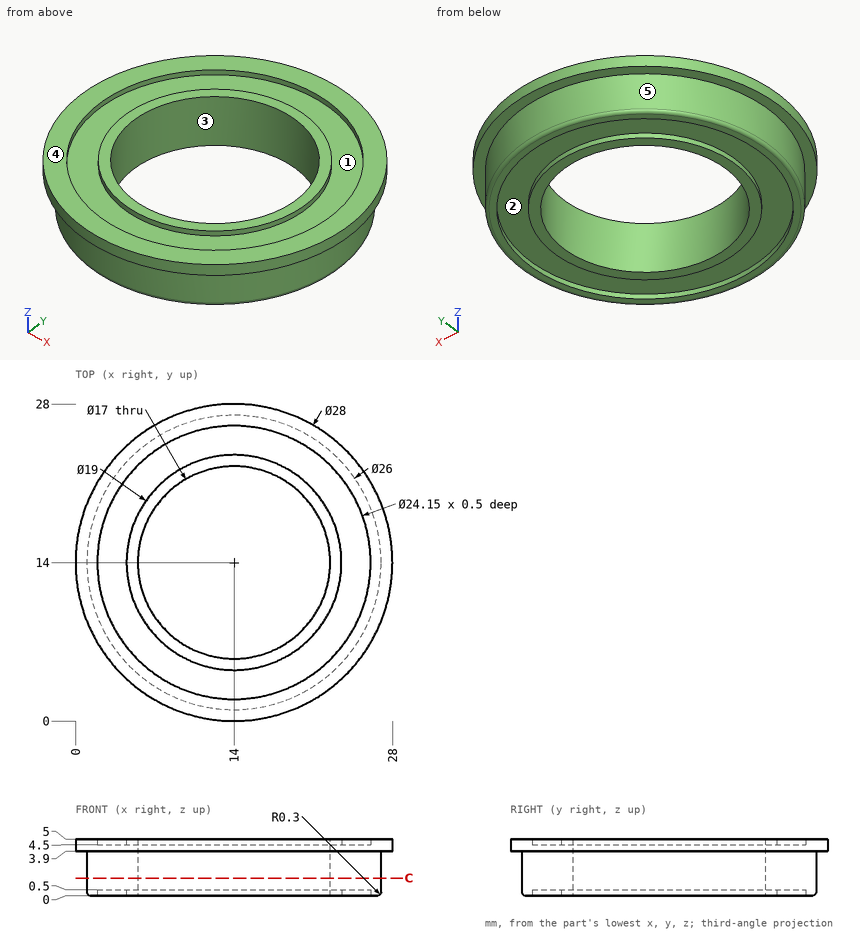
Could you check a few things on this drawing? It's one solid part, dimensions in mm from its lowest x, y, z. A direction names the side the tool comes from. Coordinates: 2 decimals unless noted, no trailing zeros. Write each loop counter-clockwise with the first axis right and the second up, starting at its lowest first coordinate (ties: lowest second). Pieces come first, ordered by that corner, then holes. Notation, with made-up numbers: (-34, 9.25) - (-9, 9.25) arc R6 ccw to (-9, 17.25) - close; hole circle Ø2 at (15, 88). An arc over 180 degrees is marked (long way). Put each result on its own line as item: value. Start each with the question number.
Q1. Thinking about a two-plate mould opening in X: for the marked faces 3, 4 and 5, which applies, pulls with the +X half, pulls with the -X half, needs draft (parallel to the pull), parting line crosses it, or undercut?
Q2. I'm going to push flat-ended pins straight in: P1, Ø1.5, axis at x = 12.5, y = 21, coming from the +Z side; P2, Ø1, axis at x = 12.5, y = 3.5, coming from the +Z side. Where does each tip first touch, or does it pass through?
Q3. Please list where these lines run through material, in increasing order: L1, parallel to Y at x = 14, z = 0.45 (3 decimals); L2, parallel to Y at x = 17.75, z = 0.3; L3, parallel to Y at x = 14, z = 2.2.
Q4. I want a section at C-C on z = 1.55. Write out the boundary of the cut face in (x, y).
Q5. Which directions (+Z, -Z, +X, -X, +Y, -Y) give clear straight access to the entire face, cutting with the end or side of a thin tool? Please do the marked faces 1 and 2.
Checks:
1. face 3: undercut
1. face 4: needs draft
1. face 5: parting line crosses it
2. P1: through
2. P2: z = 4.5
3. L1: 1 to 1.925, 4.5 to 5.5, 22.5 to 23.5, 26.075 to 27
3. L2: 1.55 to 2.52, 5.27 to 6.37, 21.63 to 22.73, 25.48 to 26.45
3. L3: 1 to 5.5, 22.5 to 27
4. outline: circle Ø26 at (14, 14); hole circle Ø17 at (14, 14)
5. face 1: +Z
5. face 2: -Z
